Can you work these out from the model? Positions are in its coordinate system, mm. A direction names the side the tool comes from. Round coordinates to 2 decimals unless told otherwise and drop trailing zeros. Loops run counter-clockwise (first coordinate to the right, second up) from the corner with the lowest first, then second, coordinate; pieces in that order, holes last. Notation, with made-up numbers: M -38.75,-15.75 L -33.75,-15.75 A24 cw -33.75,-0.75 Z; hole C 20.25,-11.5 d5. An arc over 180 degrees is marked long. Answer as CSV lines item,"result".
from build123d import *

# Parameters (mm, degrees)
F0_R     = 50
F1_DEPTH = 5


with BuildPart() as f1:
    # F0 (on Top) → F1 (new body)
    with BuildSketch(Plane.XY):
        Circle(F0_R)
        Polygon((-10, 30), (0, 30), (10, 30), (10, 10), (30, 10), (30, 0), (30, -10), (10, -10), (10, -30), (0, -30), (-10, -30), (-10, -10), (-30, -10), (-30, 0), (-30, 10), (-10, 10), align=None, mode=Mode.SUBTRACT)
    extrude(amount=F1_DEPTH)


solid = f1.part
Item 1: Will these pins go through, and if not, where does the flat tip stop? pin 1 (2.5 mm diameter, centred on y = -18, z = 3.5, fed in from -X); pin 2 (1.5 mm diameter, centred on x = -13.5, z = 1, fed in from -Y); pin 3 (2.5 mm diameter, centred on x = 24.5, z = 2.5, fed in from -Y); pin 4 (4 mm diameter, centred on x = -36.5, y = -37.5, fed in from +Z).
Output:
pin 1,"stops at x = -47.11"
pin 2,"stops at y = -48.35"
pin 3,"stops at y = -44.27"
pin 4,"passes through"
Item 2: If I drill on line 1 along Y through (x, z) = (0, 1.1); line 2 along Y through (x, z) = (-28.5, 3.55); line 3 along X through (y, z) = (-26.5, 1.8), over which ranges is the centre line in solid material (lowest first)? Write a range as from..to.
Output:
line 1,"y = -50..-30, 30..50"
line 2,"y = -41.08..-10, 10..41.08"
line 3,"x = -42.4..-10, 10..42.4"
Item 3: If we section it at A-A on y = 0: Write out the boundary of the cut face in (x, z).
Output:
outline,"M -50,0 L -30,0 L -30,5 L -50,5 Z; M 30,0 L 50,0 L 50,5 L 30,5 Z"
Item 4: If we section it at B-B on z = 2.45: Write out the boundary of the cut face in (x, y).
Output:
outline,"C 0,0 d100; hole M -30,-10 L -10,-10 L -10,-30 L 10,-30 L 10,-10 L 30,-10 L 30,10 L 10,10 L 10,30 L -10,30 L -10,10 L -30,10 Z"
Item 5: On a 3-axis mill with a long thin cutter (end or side, diameter ignored), from which of +Z, -Z, +X, -X, +Y, -Y can I reach the whole of each face in a straight line? I mean faces 1 (the face through (10.4, -10.4, 5)), 2 (the face through (-10, 20, 2)). Say none if no direction works.
Output:
face 1,"+Z, +X, -X, +Y, -Y"
face 2,"+Z, -Z"
Item 6: If we section it at D-D on x = -31.5: Write out the boundary of the cut face in (y, z), then the cut area to 3 significant figures.
Output:
outline,"M -38.83,0 L 38.83,0 L 38.83,5 L -38.83,5 Z"
area,"388 mm2"
Item 7: We'd pull the mould along Y, two halves only. Please class faces 3 (the face through (47.69, 15.02, 2.46)), 4 (the face through (-10, -20, 2)), 5 (the face through (10.4, -10.4, 0)): released by +Y, released by -Y, zero draft, split by the parting line, or undercut.
Output:
face 3,"split by the parting line"
face 4,"undercut"
face 5,"zero draft"
